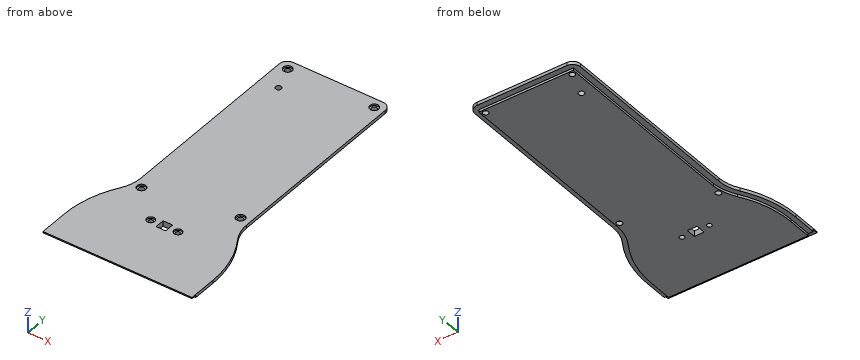
```python
from build123d import *

# Parameters (mm, degrees)
BOSS_EXTRUDE1_DEPTH = 1.5
BOSS_EXTRUDE2_DEPTH = 2
SKETCH3_W           = 1.2
SKETCH3_H           = 3.2
CUT_EXTRUDE1_DEPTH  = 210.759497368
SKETCH4_R           = 1.75
SKETCH4_R_2         = 1.5
SKETCH4_W           = 6
SKETCH4_H           = 6
CUT_EXTRUDE2_DEPTH  = 194.70221149
SKETCH5_R           = 2.75
SKETCH5_R_2         = 2.5
CUT_EXTRUDE3_DEPTH  = 1
SKETCH6_R           = 1.8
CUT_EXTRUDE4_DEPTH  = 194.70221149


with BuildPart() as part:
    # Sketch1 → Boss-Extrude1 (new body)
    with BuildSketch(Plane.XY):
        with BuildLine():
            Line((-43.5, 3.5), (-43.5, 18))
            ThreePointArc((-43.5, 18), (-41.102679313, 35.031824172), (-34.097009983, 50.740127019))
            ThreePointArc((-34.097009983, 50.740127019), (-30.928959041, 57.572199931), (-29.55199189, 64.976099479))
            Line((-29.55199189, 64.976099479), (-29.5, 65.005443368))
            Line((-29.5, 65.005443368), (-29.5, 184.505443368))
            Line((-29.5, 184.505443368), (29.5, 184.505443368))
            Line((29.5, 184.505443368), (29.5, 65.005443368))
            Line((29.5, 65.005443368), (29.55199189, 64.976099479))
            ThreePointArc((29.55199189, 64.976099479), (30.928959041, 57.572199931), (34.097009983, 50.740127019))
            ThreePointArc((34.097009983, 50.740127019), (41.102679313, 35.031824172), (43.5, 18))
            Line((43.5, 18), (43.5, 3.5))
            Line((43.5, 3.5), (-43.5, 3.5))
        make_face()
    extrude(amount=-BOSS_EXTRUDE1_DEPTH)

    # Sketch2 → Boss-Extrude2 (add)
    with BuildSketch(Plane.XY):
        with BuildLine():
            Line((-46.5, 3), (-46.5, 18))
            ThreePointArc((-46.5, 18), (-43.986116227, 35.859949502), (-36.639815607, 52.332025117))
            ThreePointArc((-36.639815607, 52.332025117), (-33.927981976, 58.412572449), (-33, 65.005443368))
            Line((-33, 65.005443368), (-33, 183.005443368))
            ThreePointArc((-33, 183.005443368), (-31.535533906, 186.540977274), (-28, 188.005443368))
            Line((-28, 188.005443368), (28, 188.005443368))
            ThreePointArc((28, 188.005443368), (31.535533906, 186.540977274), (33, 183.005443368))
            Line((33, 183.005443368), (33, 65.005443368))
            ThreePointArc((33, 65.005443368), (33.927981976, 58.412572449), (36.639815607, 52.332025117))
            ThreePointArc((36.639815607, 52.332025117), (43.986116227, 35.859949502), (46.5, 18))
            Line((46.5, 18), (46.5, 3))
            Line((46.5, 3), (46.5, 0))
            Line((46.5, 0), (-46.5, 0))
            Line((-46.5, 0), (-46.5, 3))
        make_face()
    extrude(amount=BOSS_EXTRUDE2_DEPTH)

    # Sketch3 → Cut-Extrude1 (cut, through all)
    with BuildSketch(Plane.ZY.offset(46.5)):
        with Locations((0.6, 1.6)):
            Rectangle(SKETCH3_W, SKETCH3_H)
    extrude(amount=-CUT_EXTRUDE1_DEPTH, mode=Mode.SUBTRACT)

    # Sketch4 → Cut-Extrude2 (cut, through all)
    with BuildSketch(Plane.XY.offset(2)):
        with Locations((-27, 182.005443368)):
            Circle(SKETCH4_R)
        with Locations((27, 182.005443368)):
            Circle(SKETCH4_R)
        with Locations((-28.117843442, 58.880926182)):
            Circle(SKETCH4_R)
        with Locations((27, 68.005443368)):
            Circle(SKETCH4_R)
        with Locations((-8.5, 39.912117831)):
            Circle(SKETCH4_R_2)
        with Locations((8.5, 39.912117831)):
            Circle(SKETCH4_R_2)
        with Locations((0, 39.912117831)):
            Rectangle(SKETCH4_W, SKETCH4_H)
    extrude(amount=-CUT_EXTRUDE2_DEPTH, mode=Mode.SUBTRACT)

    # Sketch5 → Cut-Extrude3 (cut)
    with BuildSketch(Plane.XY.offset(2)):
        with Locations((27, 182.005443368)):
            Circle(SKETCH5_R)
        with Locations((-27, 182.005443368)):
            Circle(SKETCH5_R)
        with Locations((-28.117843442, 58.880926182)):
            Circle(SKETCH5_R)
        with Locations((-8.5, 39.912117831)):
            Circle(SKETCH5_R_2)
        with Locations((8.5, 39.912117831)):
            Circle(SKETCH5_R_2)
        with Locations((27, 68.005443368)):
            Circle(SKETCH5_R)
    extrude(amount=-CUT_EXTRUDE3_DEPTH, mode=Mode.SUBTRACT)

    # Sketch6 → Cut-Extrude4 (cut, through all)
    with BuildSketch(Plane.XY.offset(2)):
        with Locations((-21.5, 166.615388867)):
            Circle(SKETCH6_R)
    extrude(amount=-CUT_EXTRUDE4_DEPTH, mode=Mode.SUBTRACT)


solid = part.part
```
For this review, take the finished solid that the model builds, in its own axes (mm). Coordinates: 2 decimals unless noted, no trailing zeros. Write each loop counter-clockwise with the first axis right and the second up, starting at its lowest first coordinate (ties: lowest second). Pieces come first, ordered by that corner, then holes.
(1) Wall thickness on probe 1 along Y at (x, z) = (27, -0.95); probe 2 along Y at (x, z) = (-21.5, 0.05); probe 3 along X at (y, z) = (166.5, -0.05): over which ranges is each line inside the solid? List them lowest first.
(2) For pin 1 Ø4.5 at (x, y) = (27, 182.01) entering from +Z; pin 2 Ø1 at (x, z) = (0.5, 0) entering from -Y; pin 3 Ø1.6 at (y, z) = (97.5, 1.5) entering from +X, all flat-tipped, find the tip position at first contact; note any pin that passes through.
(3) Add section C-C on x = 14.5. Give the boundary of the cut face in (y, z), then the cut area to 3 significant figures.
(4) Add section D-D on y = 30.5. Give the boundary of the cut face in (x, z).
(5) Add section B-B on y = 111. Give the boundary of the cut face in (x, z).
(6) Add section A-A on x = -21.5. Give the boundary of the cut face in (y, z).
Answer sheet:
1. probe 1: y = 3.5 to 66.26, 69.76 to 180.26, 183.76 to 184.51
1. probe 2: y = 3.2 to 164.82, 168.42 to 188.01
1. probe 3: x = -29.5 to -23.3, -19.7 to 29.5
2. pin 1: stops at z = 1
2. pin 2: stops at y = 3.2
2. pin 3: stops at x = 33
3. outline: (0, 1.2) - (3.2, 1.2) - (3.2, 0) - (3.5, 0) - (3.5, -1.5) - (184.51, -1.5) - (184.51, 0) - (188.01, 0) - (188.01, 2) - (0, 2) - close
3. area: 644 mm2
4. outline: (-45.28, 0) - (-42.22, 0) - (-42.22, -1.5) - (42.22, -1.5) - (42.22, 0) - (45.28, 0) - (45.28, 2) - (-45.28, 2) - close
5. outline: (-33, 0) - (-29.5, 0) - (-29.5, -1.5) - (29.5, -1.5) - (29.5, 0) - (33, 0) - (33, 2) - (-33, 2) - close
6. outline: (0, 1.2) - (3.2, 1.2) - (3.2, 0) - (3.5, 0) - (3.5, -1.5) - (164.82, -1.5) - (164.82, 2) - (0, 2) - close; (168.42, -1.5) - (184.51, -1.5) - (184.51, 0) - (188.01, 0) - (188.01, 2) - (168.42, 2) - close
